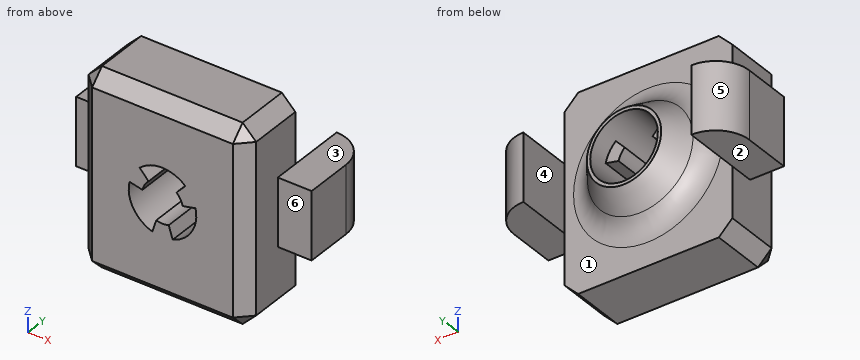
```python
from build123d import *

# Parameters (mm, degrees)
SKETCH1_W           = 24.8
SKETCH1_H           = 29
BOSS_EXTRUDE1_DEPTH = 5
SKETCH2_R           = 9
BOSS_EXTRUDE2_DEPTH = 5.8
BOSS_EXTRUDE2_TAPER = 35
SKETCH4_R           = 5
CUT_EXTRUDE2_DEPTH  = 25.771959955
BOSS_EXTRUDE3_DEPTH = 12
CHAMFER1_SIZE       = 2
FILLET2_R           = 4
SKETCH6_W           = 30
SKETCH6_H           = 2
CUT_EXTRUDE3_DEPTH  = 34.309452563
SKETCH7_W           = 10
SKETCH7_H           = 12
BOSS_EXTRUDE4_DEPTH = 5
SKETCH9_W           = 10
SKETCH9_H           = 12
BOSS_EXTRUDE5_DEPTH = 5
FILLET3_R           = 5


with BuildPart() as part:
    # Sketch1 → Boss-Extrude1 (new, symmetric)
    with BuildSketch(Plane(origin=(0, 0, 0), x_dir=(1, 0, 0), z_dir=(0, 1, 0))):
        Rectangle(SKETCH1_W, SKETCH1_H)
    extrude(amount=BOSS_EXTRUDE1_DEPTH, both=True)

    # Sketch2 → Boss-Extrude2 (add)
    with BuildSketch(Plane(origin=(0, 5, 0), x_dir=(1, 0, 0), z_dir=(0, 1, 0))):
        Circle(SKETCH2_R)
    extrude(amount=BOSS_EXTRUDE2_DEPTH, taper=BOSS_EXTRUDE2_TAPER)

    # Sketch4 → Cut-Extrude2 (cut, through all)
    with BuildSketch(Plane(origin=(0, 10.8, 0), x_dir=(1, 0, 0), z_dir=(0, 1, 0))):
        with Locations(Location((0, 0, 0), (0, 0, 270))):
            Circle(SKETCH4_R)
    extrude(amount=-CUT_EXTRUDE2_DEPTH, mode=Mode.SUBTRACT)

    # Sketch5 → Boss-Extrude3 (add)
    with BuildSketch(Plane(origin=(0, -5, 0), x_dir=(1, 0, 0), z_dir=(0, 1, 0))):
        with BuildLine():
            Line((-1.533599577, 4.863956449), (-0.917152688, 2.9088367))
            ThreePointArc((-0.917152688, 2.9088367), (0, 3.05), (0.917152688, 2.9088367))
            Line((0.917152688, 2.9088367), (1.533599577, 4.863956449))
            ThreePointArc((1.533599577, 4.863956449), (0, 5.1), (-1.533599577, 4.863956449))
        make_face()
        with BuildLine():
            Line((3.445510059, -3.760114418), (2.060550133, -2.248695877))
            ThreePointArc((2.060550133, -2.248695877), (2.641377482, -1.525), (2.977702822, -0.660140823))
            Line((2.977702822, -0.660140823), (4.979109636, -1.103842031))
            ThreePointArc((4.979109636, -1.103842031), (4.416729559, -2.55), (3.445510059, -3.760114418))
        make_face()
        with BuildLine():
            Line((-4.979109636, -1.103842031), (-2.977702822, -0.660140823))
            ThreePointArc((-2.977702822, -0.660140823), (-2.641377482, -1.525), (-2.060550133, -2.248695877))
            Line((-2.060550133, -2.248695877), (-3.445510059, -3.760114418))
            ThreePointArc((-3.445510059, -3.760114418), (-4.416729559, -2.55), (-4.979109636, -1.103842031))
        make_face()
    extrude(amount=BOSS_EXTRUDE3_DEPTH)

    # Chamfer1
    chamfer1_edges = [part.edges().sort_by_distance(p)[0] for p in [
        (0, -5, 14.5),
        (-12.4, -5, 0),
        (0, -5, -14.5),
        (12.4, -5, 0),
        (12.4, 0, 14.5),
        (-12.4, 0, 14.5),
        (-12.4, 0, -14.5),
        (12.4, 0, -14.5),
    ]]
    chamfer(chamfer1_edges, length=CHAMFER1_SIZE)

    # Fillet2
    fillet2_edges = [part.edges().sort_by_distance(p)[0] for p in [
        (-9, 5, 0),
    ]]
    fillet(fillet2_edges, radius=FILLET2_R)

    # Sketch6 → Cut-Extrude3 (cut, through all)
    with BuildSketch(Plane.XY.offset(14.5)):
        with Locations((0, 11)):
            Rectangle(SKETCH6_W, SKETCH6_H)
    extrude(amount=-CUT_EXTRUDE3_DEPTH, mode=Mode.SUBTRACT)

    # Sketch7 → Boss-Extrude4 (add)
    with BuildSketch(Plane.ZY.offset(12.4)):
        with Locations((-0.042035607, 7.386997459)):
            Rectangle(SKETCH7_W, SKETCH7_H)
    extrude(amount=BOSS_EXTRUDE4_DEPTH)

    # Sketch9 → Boss-Extrude5 (add)
    with BuildSketch(Plane(origin=(12.4, 0, 0), x_dir=(0, 0, -1), z_dir=(1, 0, 0))):
        with Locations((0.01160307, 7.425228999)):
            Rectangle(SKETCH9_W, SKETCH9_H)
    extrude(amount=BOSS_EXTRUDE5_DEPTH)

    # Fillet3
    fillet3_edges = [part.edges().sort_by_distance(p)[0] for p in [
        (17.4, 13.425228999, -0.01160307),
        (-17.4, 13.386997459, -0.042035607),
    ]]
    fillet(fillet3_edges, radius=FILLET3_R - 0.0001)  # a hair under: the kernel refuses the full size


solid = part.part
```
CAD build for the part. Positions are in the model's coordinates, mm. Face numbers are marked on the shaded views. A direction names the side the tool comes from. Coordinates: 2 decimals unless noted, no trailing zeros. Loops run counter-clockwise (first coordinate to the right, second up) from the corner with the lowest first, then second, coordinate; pieces in that order, holes last. Notation, with made-up numbers: (-32, -23.5) - (-2, -23.5) arc R36 ccw to (-2, 13.5) - close; hole circle Ø1 at (32.25, 52). An arc over 180 degrees is marked (long way). Return JSON: item names as keys, results as strings.
1. Band-saw the part on B-B (y = 7.5). Give the cut face in (x, z), and give its area (3 significant figures).
Result:
{"outline": "(-17.4, -5.04) - (-12.4, -5.04) - (-12.4, 4.96) - (-17.4, 4.96) - close; circle Ø14.5 at (0, 0); (12.4, -5.01) - (17.4, -5.01) - (17.4, 4.99) - (12.4, 4.99) - close; hole circle Ø10 at (0, 0)", "area": "187 mm2"}
2. Mould opens along X. For the marked faces 4, 5 and 6 say: released by +X, released by -X, zero draft, split by the parting line, or undercut.
Result:
{"face 4": "undercut", "face 5": "released by -X", "face 6": "zero draft"}
3. 3-axis set-ups, long thin cutter, end or side, ignore diameter. For the marked faces 1, 2 and 3: which of +Z, -Z, +X, -X, +Y, -Y reach the whole face in a straight line?
Result:
{"face 1": "+Y", "face 2": "-Z, -X, +Y, -Y", "face 3": "+Z, +X, +Y, -Y"}
4. Band-saw the part on D-D (y = 12). Give the cut face in (x, z), and give its area (3 significant figures).
Result:
{"outline": "(-15.86, -5.04) - (-12.4, -5.04) - (-12.4, 4.96) - (-15.86, 4.96) - close; (12.4, -5.01) - (15.9, -5.01) - (15.9, 4.99) - (12.4, 4.99) - close", "area": "69.5 mm2"}
5. Band-saw the part on A-A (x = 0). Give the cut face in (y, z), and give its area (3 significant figures).
Result:
{"outline": "(-5, -12.5) - (-3, -14.5) - (5, -14.5) - (5, -11.08) arc R4 cw to (6.71, -7.81) - (10, -5.5) - (10, -5) - (7, -5) - (7, -3.05) - (-5, -3.05) - close; (-5, 5) - (10, 5) - (10, 5.5) - (6.71, 7.81) arc R4 cw to (5, 11.08) - (5, 14.5) - (-3, 14.5) - (-5, 12.5) - close", "area": "233 mm2"}
6. Band-saw the part on C-C (y = -3.5). Give the cut face in (x, z).
Result:
{"outline": "(-11.9, -12.5) - (-10.4, -14) - (10.4, -14) - (11.9, -12.5) - (11.9, 12.5) - (10.4, 14) - (-10.4, 14) - (-11.9, 12.5) - close; hole (-4.88, 1.08) arc R5 ccw to (-1.5, -4.77) - (-0.92, -2.91) arc R3.05 ccw to (0.92, -2.91) - (1.5, -4.77) arc R5 ccw to (4.88, 1.08) - (2.98, 0.66) arc R3.05 ccw to (2.06, 2.25) - (3.38, 3.69) arc R5 ccw to (-3.38, 3.69) - (-2.06, 2.25) arc R3.05 ccw to (-2.98, 0.66) - close"}
7. Drop flat-ended pins along their axis: pin 1 (1.5 mm diameter, centred on x = 14.5, z = -2, fed in from -Y); pin 2 (2.5 mm diameter, centred on x = -0.5, z = -4, fed in from +Y); pin 3 (4 mm diameter, centred on x = 13.5, y = 4, fed in from -Z). Give the stop position or say it passes through.
Result:
{"pin 1": "stops at y = 1.43", "pin 2": "stops at y = 10", "pin 3": "stops at z = -13.4"}
8. Probe L1, parallel to Z at x = 0, y = -0.5; L2, parallel to X at y = 3.5, z = 0; L3, parallel to Z at x = -14, y = 12. List the from-to ranges inside material, lowest first. Write a range as from..to.
Result:
{"L1": "z = -14.5..-3.05, 5..14.5", "L2": "x = -17.4..-5, 5..17.4", "L3": "z = -5.04..4.96"}
